Can you work these out from the model? Positions are in its coordinate system, mm. Face numbers are marked on the shaded views. A direction names the side the tool comes from. Give positions to 0.01 mm unless a question says otherwise; leave off trailing zeros. Order: outer loops, then holes, each group sorted by start corner. A loop starts at its lowest first (then second) coordinate and runs counter-clockwise, first axis right, second up. Notation, with made-up numbers: (87.5, 31.25) -> (144.5, 31.25) arc R18 ccw to (144.5, 55.25) -> close; hole circle Ø4 at (-36, -26.5). An arc over 180 degrees is marked (long way). Answer as a JSON object with one key per item and string values.
```python
from build123d import *

# Parameters (mm, degrees)
SKETCH1_W           = 104
SKETCH1_H           = 154
SKETCH1_W_2         = 100
SKETCH1_H_2         = 150
BOSS_EXTRUDE1_DEPTH = 30
SKETCH1_2_W         = 104
SKETCH1_2_H         = 154
SKETCH1_2_W_2       = 100
SKETCH1_2_H_2       = 150
BOSS_EXTRUDE2_DEPTH = 2
FILLET1_R           = 3
SKETCH2_R           = 2.075
BOSS_EXTRUDE3_DEPTH = 2
SKETCH3_R           = 2.075
BOSS_EXTRUDE4_DEPTH = 2
SKETCH4_R           = 5
CUT_EXTRUDE1_DEPTH  = 10
FILLET2_R           = 0.5
FILLET3_R           = 2


with BuildPart() as part:
    # Sketch1 → Boss-Extrude1 (new body)
    with BuildSketch(Plane(origin=(0, 0, 0), x_dir=(1, 0, 0), z_dir=(0, 1, 0))):
        Rectangle(SKETCH1_W, SKETCH1_H)
        Rectangle(SKETCH1_W_2, SKETCH1_H_2, mode=Mode.SUBTRACT)
    extrude(amount=BOSS_EXTRUDE1_DEPTH)

    # Sketch1_2 → Boss-Extrude2 (add)
    # profile 1 of 2: a face of its own
    with BuildSketch(Plane(origin=(0, 0, 0), x_dir=(1, 0, 0), z_dir=(0, 1, 0))):
        Rectangle(SKETCH1_2_W, SKETCH1_2_H)
        Rectangle(SKETCH1_2_W_2, SKETCH1_2_H_2, mode=Mode.SUBTRACT)
    # profile 2 of 2: a face of its own
    with BuildSketch(Plane(origin=(0, 0, 0), x_dir=(1, 0, 0), z_dir=(0, 1, 0))):
        Rectangle(SKETCH1_2_W_2, SKETCH1_2_H_2)
    extrude(amount=-BOSS_EXTRUDE2_DEPTH)

    # Fillet1
    fillet1_edges = [part.edges().sort_by_distance(p)[0] for p in [
        (50, 15, 75),
        (50, 15, -75),
        (-50, 15, -75),
        (-50, 15, 75),
        (-52, 14, -77),
        (52, 14, -77),
        (52, 14, 77),
        (-52, 14, 77),
    ]]
    fillet(fillet1_edges, radius=FILLET1_R)

    # Sketch2 → Boss-Extrude3 (add)
    with BuildSketch(Plane(origin=(0, 30, 0), x_dir=(1, 0, 0), z_dir=(0, 1, 0))):
        with BuildLine():
            Line((56.25, 68.25), (52, 68.25))
            Line((52, 68.25), (52, 59.75))
            Line((52, 59.75), (56.25, 59.75))
            ThreePointArc((56.25, 59.75), (60.5, 64), (56.25, 68.25))
        make_face()
        with Locations(Location((56.25, 64, 0), (0, 0, 270))):
            Circle(SKETCH2_R, mode=Mode.SUBTRACT)
    extrude(amount=-BOSS_EXTRUDE3_DEPTH)

    # Sketch3 → Boss-Extrude4 (add)
    with BuildSketch(Plane(origin=(0, 30, 0), x_dir=(1, 0, 0), z_dir=(0, 1, 0))):
        with BuildLine():
            Line((-52, -59.75), (-56.25, -59.75))
            ThreePointArc((-56.25, -59.75), (-60.5, -64), (-56.25, -68.25))
            Line((-56.25, -68.25), (-52, -68.25))
            Line((-52, -68.25), (-52, -59.75))
        make_face()
        with Locations(Location((-56.25, -64, 0), (0, 0, 270))):
            Circle(SKETCH3_R, mode=Mode.SUBTRACT)
    extrude(amount=-BOSS_EXTRUDE4_DEPTH)

    # Sketch4 → Cut-Extrude1 (cut)
    with BuildSketch(Plane(origin=(0, 0, -77), x_dir=(-1, 0, 0), z_dir=(0, 0, -1))):
        with Locations((0, 20)):
            Circle(SKETCH4_R)
    extrude(amount=-CUT_EXTRUDE1_DEPTH, mode=Mode.SUBTRACT)

    # Fillet2
    fillet2_edges = [part.edges().sort_by_distance(p)[0] for p in [
        (5, 20, -75),
        (5, 20, -77),
    ]]
    fillet(fillet2_edges, radius=FILLET2_R)

    # Fillet3
    fillet3_edges = [part.edges().sort_by_distance(p)[0] for p in [
        (52, 29, -59.75),
        (52, 29, -68.25),
        (-52, 29, 59.75),
        (-52, 29, 68.25),
    ]]
    fillet(fillet3_edges, radius=FILLET3_R)


solid = part.part
```
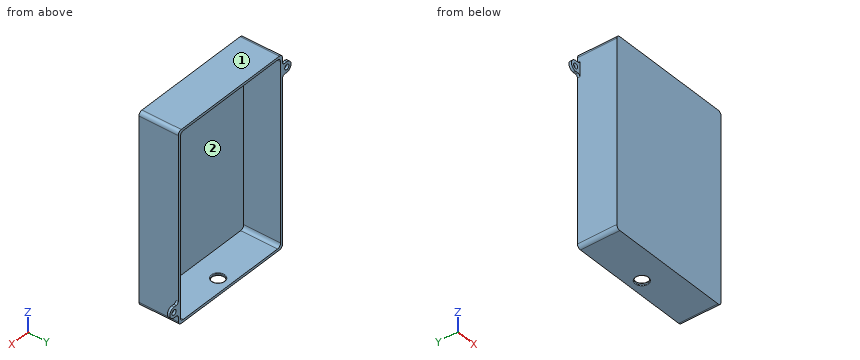
1. If we section it at B-B on x = 0: Please give me the cut outline in (y, z), then the cut area to 3 significant figures.
Worked answers:
{"outline": "(-2, -77) -> (14.5, -77) arc R0.5 ccw to (15, -76.5) -> (15, -75.5) arc R0.5 ccw to (14.5, -75) -> (0, -75) -> (0, 75) -> (30, 75) -> (30, 77) -> (-2, 77) -> close; (25, -76.5) arc R0.5 ccw to (25.5, -77) -> (30, -77) -> (30, -75) -> (25.5, -75) arc R0.5 ccw to (25, -75.5) -> close", "area": "408 mm²"}
2. If we section it at A-A on z = 64: Please give me the cut outline in (x, y) (3 decimals).
Worked answers:
{"outline": "(-60.5, 28) -> (-58.325, 28) -> (-58.325, 30) -> (-60.5, 30) -> close; (-54.175, 28) -> (-52, 28) -> (-52, -2) -> (52, -2) -> (52, 30) -> (50, 30) -> (50, 0) -> (-50, 0) -> (-50, 30) -> (-54.175, 30) -> close"}
3. If we section it at C-C on y = 3: Please give me the cut outline in (x, z).
Worked answers:
{"outline": "(-52, -74) arc R3 ccw to (-49, -77) -> (49, -77) arc R3 ccw to (52, -74) -> (52, 74) arc R3 ccw to (49, 77) -> (-49, 77) arc R3 ccw to (-52, 74) -> close; hole (-50, -72) arc R3 ccw to (-47, -75) -> (47, -75) arc R3 ccw to (50, -72) -> (50, 72) arc R3 ccw to (47, 75) -> (-47, 75) arc R3 ccw to (-50, 72) -> close"}
4. Please list where these lines run through material, in increasing order: L1, parallel to X at y = 28.65, z = 64 (3 decimals); L2, parallel to X at y = 28.7, z = -64 (3 decimals); L3, parallel to X at y = 28, z = 44.
Worked answers:
{"L1": "-60.5 to -58.325, -54.175 to -50, 50 to 52", "L2": "-52 to -50, 50 to 54.175, 58.325 to 60.5", "L3": "-52 to -50, 50 to 52"}
5. For the marked faces 1 and 2, which set-ups out of +Z, -Z, +X, -X, +Y, -Y let a thin tool reach every point of the face, with its end or its side?
Worked answers:
{"face 1": "+Z, +X, -X, +Y, -Y", "face 2": "+Y"}
6. Will these pins go through, and if not, where does the flat tip stop? pin 1 Ø5.5 at (x, z) = (56.25, -64) entering from +Y; pin 2 Ø12 at (y, z) = (20, -39) entering from +X; pin 3 Ø1 at (x, y) = (-55.5, 28.5) entering from -Z; pin 4 Ø12 at (x, z) = (13, -60.5) entering from +Y.
Worked answers:
{"pin 1": "y = 30", "pin 2": "x = 52", "pin 3": "z = 59.75", "pin 4": "y = 0"}
7. If we section it at D-D on x = -29: Please give me the cut outline in (y, z).
Worked answers:
{"outline": "(-2, -77) -> (30, -77) -> (30, -75) -> (0, -75) -> (0, 75) -> (30, 75) -> (30, 77) -> (-2, 77) -> close"}
